Can you work these out from the drawing? Everything is in mm from the part's minimum corner. A direction names the side the tool comes from. Give positions to 0.01 mm unless a question says otherwise; leave off trailing zeros. Order: outer loops, then holes, each group sorted by start corner. A loop starts at its lowest first (then second) coordinate and runs counter-clockwise, first axis right, second up. Notation, with made-up numbers: (57, 2) - (110, 2) arc R21 ccw to (110, 7) - close; hole circle Ø6 at (71.25, 30). An arc over 180 degrees is marked (long way). One line per question, with ' | ' between items.
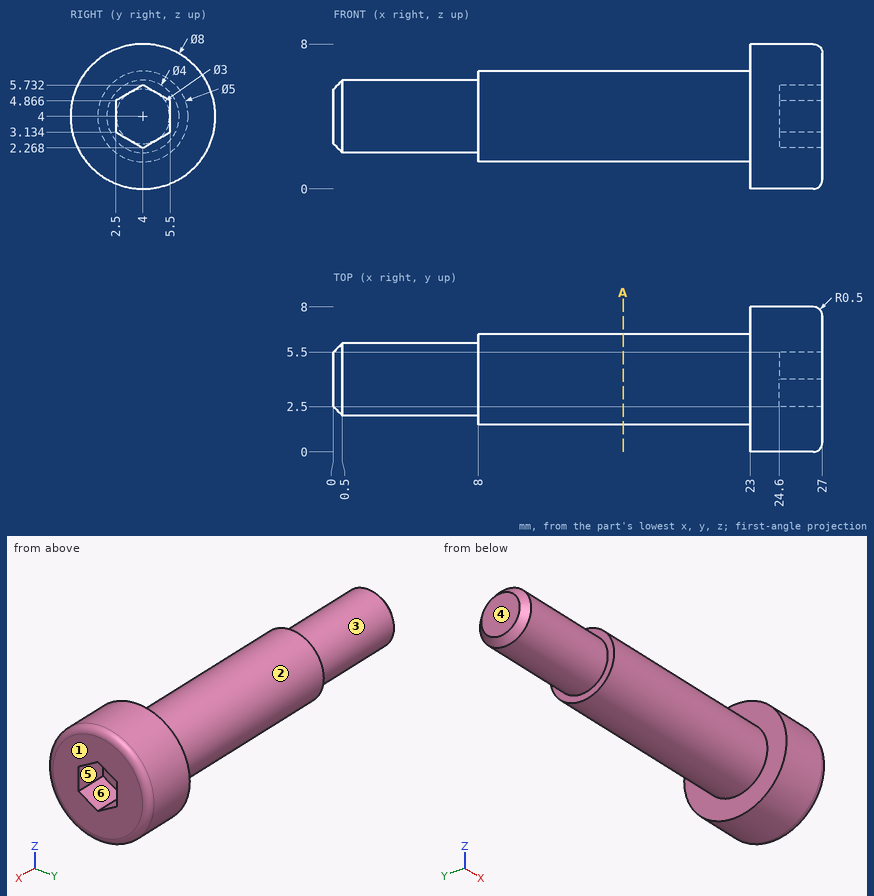
1) I want a section at A-A (x = 16). List the corners of the cut face in (y, z) for me, plus the area to 3 significant figures.
Model answer:
outline: circle Ø5 at (4, 4) | area: 19.6 mm2
2) Thinking about a two-plate mould opening in Y: for the marked faces 3, 4, 5 and 6, which applies, +Y half, -Y half, draft (parallel to the pull), parting line (faces both ways), or undercut?
Model answer:
face 3: parting line | face 4: draft | face 5: undercut | face 6: undercut
3) Please list where these lines run through material, in increasing order: L1, parallel to Z at x = 13, y = 2; L2, parallel to X at y = 6.25, z = 5; L3, parallel to Y at x = 16.75, z = 2.5.
Model answer:
L1: z = 2.5 to 5.5 | L2: x = 8 to 27 | L3: y = 2 to 6
4) On a 3-axis mill with a long thin cutter (end or side, diameter ignored), from which of +Z, -Z, +X, -X, +Y, -Y can I reach the whole of each face in a straight line? I mean the marked faces 1 and 2. Say none if no direction works.
Model answer:
face 1: +Z, -Z, +X, +Y, -Y | face 2: -X
5) I'm going to push flat-ended pins straight in: P1, Ø1, axis at y = 5, z = 4, coming from the -X side; P2, Ø1.5, axis at y = 1.5, z = 6, coming from the -X side; P3, Ø1, axis at x = 14, y = 4.5, coming from the +Z side. Where does each tip first touch, or does it pass through?
Model answer:
P1: stops at x = 0 | P2: stops at x = 8 | P3: stops at z = 6.5
